Build history of the part. All positions in model axes, mm. A direction names the side the tool comes from. Coordinates: 2 decimals unless noted, no trailing zeros. Loops run counter-clockwise (first coordinate to the right, second up) from the corner with the lowest first, then second, coordinate; pieces in that order, holes last.
Item 1: Cut at B-B (x = -7.65). List the corners of the cut face in (y, z).
Item 2: Mould opens along Y. For faces 3 (the face through (5, 10, 0)), 4 (the face through (0, 0, 0)), 5 (the face through (10.25, 1, 0)) say: released by +Y, released by -Y, zero draft, split by the parting line, or undercut.
Item 3: Cut at C-C (x = 5). List the corners of the cut face in (y, z), and give its area (3 significant figures).
Item 4: Cut at D-D (y = 5.5). List the corners of the cut face in (x, z).
Item 5: Drill centre lines: line 1 along X through (y, z) = (1.3, 10.35); line 2 along Z through (x, y) = (7.65, 1.05); line 3 along Y through (x, z) = (2.5, -7). Where is each one in solid material? Low to high.
Item 6: Flat gauge pins, fed straight in: pin 1 (3.5 mm diameter, centred on x = -7.65, z = 10.35, fed in from +Y); pin 2 (1.5 mm diameter, centred on x = -1.5, z = -8, fed in from -Y); pin 3 (4 mm diameter, centred on y = 7.5, z = 5.5, fed in from +X). Where does each tip first touch, or does it go through?
Item 7: Cut at A-A (z = 10.35). List the corners of the cut face in (x, y).
Item 8: 3-axis set-ups, long thin cutter, end or side, ignore diameter. For faces 1 (the face through (8.1, 5.94, -0.98)), 2 (the face through (0, 1, -12.5)): which of +Z, -Z, +X, -X, +Y, -Y reach the whole face in a straight line?
from build123d import *

# Parameters (mm, degrees)
SKETCH1_W           = 20.5
SKETCH1_H           = 25
BOSS_EXTRUDE1_DEPTH = 2
SKETCH2_R           = 1.15
CUT_EXTRUDE1_DEPTH  = 3
SKETCH3_R           = 3.25
BOSS_EXTRUDE2_DEPTH = 8


with BuildPart() as part:
    # Sketch1 → Boss-Extrude1 (new body)
    with BuildSketch(Plane(origin=(0, 0, 0), x_dir=(1, 0, 0), z_dir=(0, 1, 0))):
        Rectangle(SKETCH1_W, SKETCH1_H)
    extrude(amount=BOSS_EXTRUDE1_DEPTH)

    # Sketch2 → Cut-Extrude1 (cut, through all)
    with BuildSketch(Plane(origin=(0, 2, 0), x_dir=(1, 0, 0), z_dir=(0, 1, 0))):
        with Locations((7.65, -10.35)):
            Circle(SKETCH2_R)
        with Locations((-7.65, -10.35)):
            Circle(SKETCH2_R)
    extrude(amount=-CUT_EXTRUDE1_DEPTH, mode=Mode.SUBTRACT)

    # Sketch3 → Boss-Extrude2 (add)
    with BuildSketch(Plane(origin=(0, 2, 0), x_dir=(1, 0, 0), z_dir=(0, 1, 0))):
        with Locations((5, 0)):
            Circle(SKETCH3_R)
    extrude(amount=BOSS_EXTRUDE2_DEPTH)


solid = part.part
Filled sheet:
1. outline: (0, -12.5) - (2, -12.5) - (2, 9.2) - (0, 9.2) - close; (0, 11.5) - (2, 11.5) - (2, 12.5) - (0, 12.5) - close
2. face 3: released by +Y
2. face 4: released by -Y
2. face 5: zero draft
3. outline: (0, -12.5) - (2, -12.5) - (2, -3.25) - (10, -3.25) - (10, 3.25) - (2, 3.25) - (2, 12.5) - (0, 12.5) - close
3. area: 102 mm2
4. outline: circle Ø6.5 at (5, 0)
5. line 1: x = -10.25 to -8.8, -6.5 to 6.5, 8.8 to 10.25
5. line 2: z = -12.5 to 9.2, 11.5 to 12.5
5. line 3: y = 0 to 2
6. pin 1: stops at y = 2
6. pin 2: stops at y = 0
6. pin 3: passes through
7. outline: (-10.25, 0) - (-8.8, 0) - (-8.8, 2) - (-10.25, 2) - close; (-6.5, 0) - (6.5, 0) - (6.5, 2) - (-6.5, 2) - close; (8.8, 0) - (10.25, 0) - (10.25, 2) - (8.8, 2) - close
8. face 1: +Y
8. face 2: -Z, +X, -X, +Y, -Y
